from build123d import *

# Parameters (mm, degrees)
SKETCH_1_W          = 25
SKETCH_1_H          = 5
SKETCH_1_W_2        = 70
SKETCH_1_H_2        = 190
EXTRUDE_1_DEPTH     = 5
SKETCH_3_W          = 50
SKETCH_3_H          = 67.5
CUT_EXTRUDE_2_DEPTH = 5
FILLET_1_R          = 10
CUT_EXTRUDE_3_DEPTH = 10
SKETCH_6_W          = 5
SKETCH_6_H          = 220
EXTRUDE_2_DEPTH     = 5
MOVE_FACE_1_DEPTH   = 5
FILLET_2_R          = 10


# Read off the part's stored shape, not the designer's step: 移动面1
with BuildPart() as part:
    # 草图1 → 凸台-拉伸1 (new body)
    with BuildSketch(Plane.XY):
        with Locations((57.5, 192.5)):
            Rectangle(SKETCH_1_W, SKETCH_1_H)
        with Locations((35, 95)):
            Rectangle(SKETCH_1_W_2, SKETCH_1_H_2)
        with Locations((12.5, 192.5)):
            Rectangle(SKETCH_1_W, SKETCH_1_H)
        with Locations((57.5, -2.5)):
            Rectangle(SKETCH_1_W, SKETCH_1_H)
        with Locations((12.5, -2.5)):
            Rectangle(SKETCH_1_W, SKETCH_1_H)
        Polygon((25, -5), (0, -5), (0, -15), (70, -15), (70, -5), (45, -5), (45, 0), (25, 0), align=None)
        Polygon((25, 195), (25, 190), (45, 190), (45, 195), (70, 195), (70, 205), (0, 205), (0, 195), align=None)
    extrude(amount=EXTRUDE_1_DEPTH)

    # 草图3 → 切除-拉伸2 (cut)
    with BuildSketch(Plane.XY.offset(5)):
        with Locations((35, 53.75)):
            Rectangle(SKETCH_3_W, SKETCH_3_H)
        with Locations((35, 136.25)):
            Rectangle(SKETCH_3_W, SKETCH_3_H)
    extrude(amount=-CUT_EXTRUDE_2_DEPTH, mode=Mode.SUBTRACT)

    # 圆角1
    fillet_1_edges = [part.edges().sort_by_distance(p)[0] for p in [
        (10, 20, 2.5),
        (10, 87.5, 2.5),
        (60, 87.5, 2.5),
        (60, 20, 2.5),
        (10, 102.5, 2.5),
        (10, 170, 2.5),
        (60, 170, 2.5),
        (60, 102.5, 2.5),
    ]]
    fillet(fillet_1_edges, radius=FILLET_1_R)

    # 草图5 → 切除-拉伸3 (cut)
    with BuildSketch(Plane.XY.offset(5)):
        with BuildLine():
            Line((3.1, 0), (21.9, 0))
            ThreePointArc((21.9, 0), (23.45, 1.55), (25, 0))
            Line((25, 0), (25, -5))
            ThreePointArc((25, -5), (23.45, -6.55), (21.9, -5))
            Line((21.9, -5), (3.1, -5))
            ThreePointArc((3.1, -5), (1.55, -6.55), (0, -5))
            Line((0, -5), (0, 0))
            ThreePointArc((0, 0), (1.55, 1.55), (3.1, 0))
        make_face()
        with BuildLine():
            Line((45, 0), (45, -5))
            ThreePointArc((45, -5), (46.55, -6.55), (48.1, -5))
            Line((48.1, -5), (66.9, -5))
            ThreePointArc((66.9, -5), (68.45, -6.55), (70, -5))
            Line((70, -5), (70, 0))
            ThreePointArc((70, 0), (68.45, 1.55), (66.9, 0))
            Line((66.9, 0), (48.1, 0))
            ThreePointArc((48.1, 0), (46.55, 1.55), (45, 0))
        make_face()
        with BuildLine():
            Line((66.9, 190), (48.1, 190))
            ThreePointArc((48.1, 190), (46.55, 188.45), (45, 190))
            Line((45, 190), (45, 195))
            ThreePointArc((45, 195), (46.55, 196.55), (48.1, 195))
            Line((48.1, 195), (66.9, 195))
            ThreePointArc((66.9, 195), (68.45, 196.55), (70, 195))
            Line((70, 195), (70, 190))
            ThreePointArc((70, 190), (68.45, 188.45), (66.9, 190))
        make_face()
        with BuildLine():
            Line((25, 190), (25, 195))
            ThreePointArc((25, 195), (23.45, 196.55), (21.9, 195))
            Line((21.9, 195), (3.1, 195))
            ThreePointArc((3.1, 195), (1.55, 196.55), (0, 195))
            Line((0, 195), (0, 190))
            ThreePointArc((0, 190), (1.55, 188.45), (3.1, 190))
            Line((3.1, 190), (21.9, 190))
            ThreePointArc((21.9, 190), (23.45, 188.45), (25, 190))
        make_face()
    extrude(amount=-CUT_EXTRUDE_3_DEPTH, mode=Mode.SUBTRACT)

    # 草图6 → 凸台-拉伸2 (add)
    with BuildSketch(Plane.XY.offset(5)):
        with Locations((72.5, 95)):
            Rectangle(SKETCH_6_W, SKETCH_6_H)
        with Locations((-2.5, 95)):
            Rectangle(SKETCH_6_W, SKETCH_6_H)
    extrude(amount=-EXTRUDE_2_DEPTH)

    # Move Face 1 outline → Move Face 1 (cut)
    # profile 1 of 4: a face of its own
    with BuildSketch(Plane.XY):
        with BuildLine():
            Line((21.850781441, 0.05), (3.149218559, 0.05))
            ThreePointArc((3.149218559, 0.05), (1.524996947, 1.599804628), (-0.05, 0))
            Line((-0.05, 0), (-0.05, -5))
            ThreePointArc((-0.05, -5), (1.524996947, -6.599804628), (3.149218559, -5.05))
            Line((3.149218559, -5.05), (21.850781441, -5.05))
            ThreePointArc((21.850781441, -5.05), (23.475003053, -6.599804628), (25.05, -5))
            Line((25.05, -5), (25.05, 0))
            ThreePointArc((25.05, 0), (23.475003053, 1.599804628), (21.850781441, 0.05))
        make_face()
        with BuildLine():
            ThreePointArc((0, 0), (1.55, 1.55), (3.1, 0))
            Line((3.1, 0), (21.9, 0))
            ThreePointArc((21.9, 0), (23.45, 1.55), (25, 0))
            Line((25, 0), (25, -5))
            ThreePointArc((25, -5), (23.45, -6.55), (21.9, -5))
            Line((21.9, -5), (3.1, -5))
            ThreePointArc((3.1, -5), (1.55, -6.55), (0, -5))
            Line((0, -5), (0, 0))
        make_face(mode=Mode.SUBTRACT)
    # profile 2 of 4: a face of its own
    with BuildSketch(Plane.XY):
        with BuildLine():
            ThreePointArc((70.05, 0), (68.475003053, 1.599804628), (66.850781441, 0.05))
            Line((66.850781441, 0.05), (48.149218559, 0.05))
            ThreePointArc((48.149218559, 0.05), (46.524996947, 1.599804628), (44.95, 0))
            Line((44.95, 0), (44.95, -5))
            ThreePointArc((44.95, -5), (46.524996947, -6.599804628), (48.149218559, -5.05))
            Line((48.149218559, -5.05), (66.850781441, -5.05))
            ThreePointArc((66.850781441, -5.05), (68.475003053, -6.599804628), (70.05, -5))
            Line((70.05, -5), (70.05, 0))
        make_face()
        with BuildLine():
            Line((48.1, 0), (66.9, 0))
            ThreePointArc((66.9, 0), (68.45, 1.55), (70, 0))
            Line((70, 0), (70, -5))
            ThreePointArc((70, -5), (68.45, -6.55), (66.9, -5))
            Line((66.9, -5), (48.1, -5))
            ThreePointArc((48.1, -5), (46.55, -6.55), (45, -5))
            Line((45, -5), (45, 0))
            ThreePointArc((45, 0), (46.55, 1.55), (48.1, 0))
        make_face(mode=Mode.SUBTRACT)
    # profile 3 of 4: a face of its own
    with BuildSketch(Plane.XY):
        with BuildLine():
            ThreePointArc((21.850781441, 189.95), (23.475003053, 188.400195372), (25.05, 190))
            Line((25.05, 190), (25.05, 195))
            ThreePointArc((25.05, 195), (23.475003053, 196.599804628), (21.850781441, 195.05))
            Line((21.850781441, 195.05), (3.149218559, 195.05))
            ThreePointArc((3.149218559, 195.05), (1.524996947, 196.599804628), (-0.05, 195))
            Line((-0.05, 195), (-0.05, 190))
            ThreePointArc((-0.05, 190), (1.524996947, 188.400195372), (3.149218559, 189.95))
            Line((3.149218559, 189.95), (21.850781441, 189.95))
        make_face()
        with BuildLine():
            Line((25, 195), (25, 190))
            ThreePointArc((25, 190), (23.45, 188.45), (21.9, 190))
            Line((21.9, 190), (3.1, 190))
            ThreePointArc((3.1, 190), (1.55, 188.45), (0, 190))
            Line((0, 190), (0, 195))
            ThreePointArc((0, 195), (1.55, 196.55), (3.1, 195))
            Line((3.1, 195), (21.9, 195))
            ThreePointArc((21.9, 195), (23.45, 196.55), (25, 195))
        make_face(mode=Mode.SUBTRACT)
    # profile 4 of 4: a face of its own
    with BuildSketch(Plane.XY):
        with BuildLine():
            ThreePointArc((48.149218559, 195.05), (46.524996947, 196.599804628), (44.95, 195))
            Line((44.95, 195), (44.95, 190))
            ThreePointArc((44.95, 190), (46.524996947, 188.400195372), (48.149218559, 189.95))
            Line((48.149218559, 189.95), (66.850781441, 189.95))
            ThreePointArc((66.850781441, 189.95), (68.475003053, 188.400195372), (70.05, 190))
            Line((70.05, 190), (70.05, 195))
            ThreePointArc((70.05, 195), (68.475003053, 196.599804628), (66.850781441, 195.05))
            Line((66.850781441, 195.05), (48.149218559, 195.05))
        make_face()
        with BuildLine():
            Line((45, 190), (45, 195))
            ThreePointArc((45, 195), (46.55, 196.55), (48.1, 195))
            Line((48.1, 195), (66.9, 195))
            ThreePointArc((66.9, 195), (68.45, 196.55), (70, 195))
            Line((70, 195), (70, 190))
            ThreePointArc((70, 190), (68.45, 188.45), (66.9, 190))
            Line((66.9, 190), (48.1, 190))
            ThreePointArc((48.1, 190), (46.55, 188.45), (45, 190))
        make_face(mode=Mode.SUBTRACT)
    extrude(amount=MOVE_FACE_1_DEPTH, mode=Mode.SUBTRACT)

    # 圆角2
    fillet_2_edges = [part.edges().sort_by_distance(p)[0] for p in [
        (75, 205, 2.5),
        (75, -15, 2.5),
        (-5, -15, 2.5),
        (-5, 205, 2.5),
    ]]
    fillet(fillet_2_edges, radius=FILLET_2_R)


solid = part.part
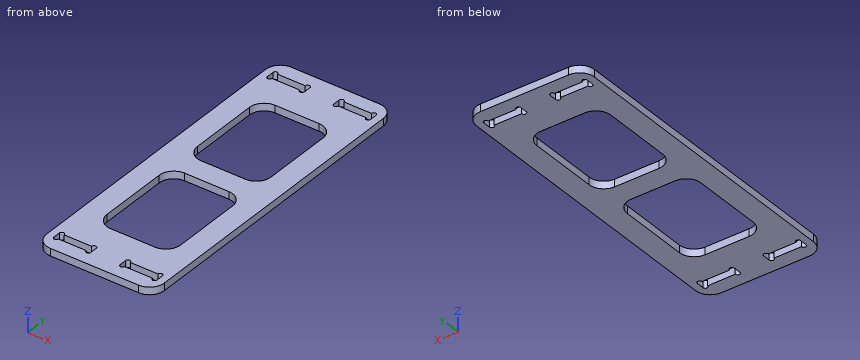
Geometry: final body of the model. Coordinates: model frame, mm. Give positions to 0.01 mm unless a question says otherwise; leave off trailing zeros. Loops run counter-clockwise (first coordinate to the right, second up) from the corner with the lowest first, then second, coordinate; pieces in that order, holes last. Notation, with made-up numbers: (71.25, 56) - (104.25, 56) arc R4 ccw to (104.25, 63) - close; hole circle Ø10 at (66, -23). An arc over 180 degrees is marked (long way). One line per question, with ' | ' between items. Start each with the question number.
(1) Ray query, line 1 (Y direction, x = 62, z = 1.95); line 2 (Y direction, x = 35, z = 1.35); line 3 (X direction, y = 56, z = 2.05). Return the intervals inside material, ascending. Write a range as from..to.
(2) Section query C-C on x = 40. Return loops of the section in (y, z).
(3) Section query A-A on x = 56. Return loops of the section in (y, z), then the cut area to 3 significant figures.
(4) Section query D-D on z = 2.75. Count the separate pieces of the cut face and the enclosed holes in it, then the cut area to 3 significant figures.
(5) Section query B-B on y = 142. Return loops of the section in (x, z).
The answers:
1) line 1: -15..-5.05, 0.05..189.95, 195.05..205 | line 2: -15..20, 87.5..102.5, 170..205 | line 3: -5..10, 60..75
2) outline: (-15, 0) - (20, 0) - (20, 5) - (-15, 5) - close; (87.5, 0) - (102.5, 0) - (102.5, 5) - (87.5, 5) - close; (170, 0) - (205, 0) - (205, 5) - (170, 5) - close
3) outline: (-15, 0) - (-5.05, 0) - (-5.05, 5) - (-15, 5) - close; (0.05, 0) - (22, 0) - (22, 5) - (0.05, 5) - close; (85.5, 0) - (104.5, 0) - (104.5, 5) - (85.5, 5) - close; (168, 0) - (189.95, 0) - (189.95, 5) - (168, 5) - close; (195.05, 0) - (205, 0) - (205, 5) - (195.05, 5) - close | area: 414 mm2
4) separate pieces: 1 | enclosed holes: 6 | area: 10,400 mm2
5) outline: (-5, 0) - (10, 0) - (10, 5) - (-5, 5) - close; (60, 0) - (75, 0) - (75, 5) - (60, 5) - close
